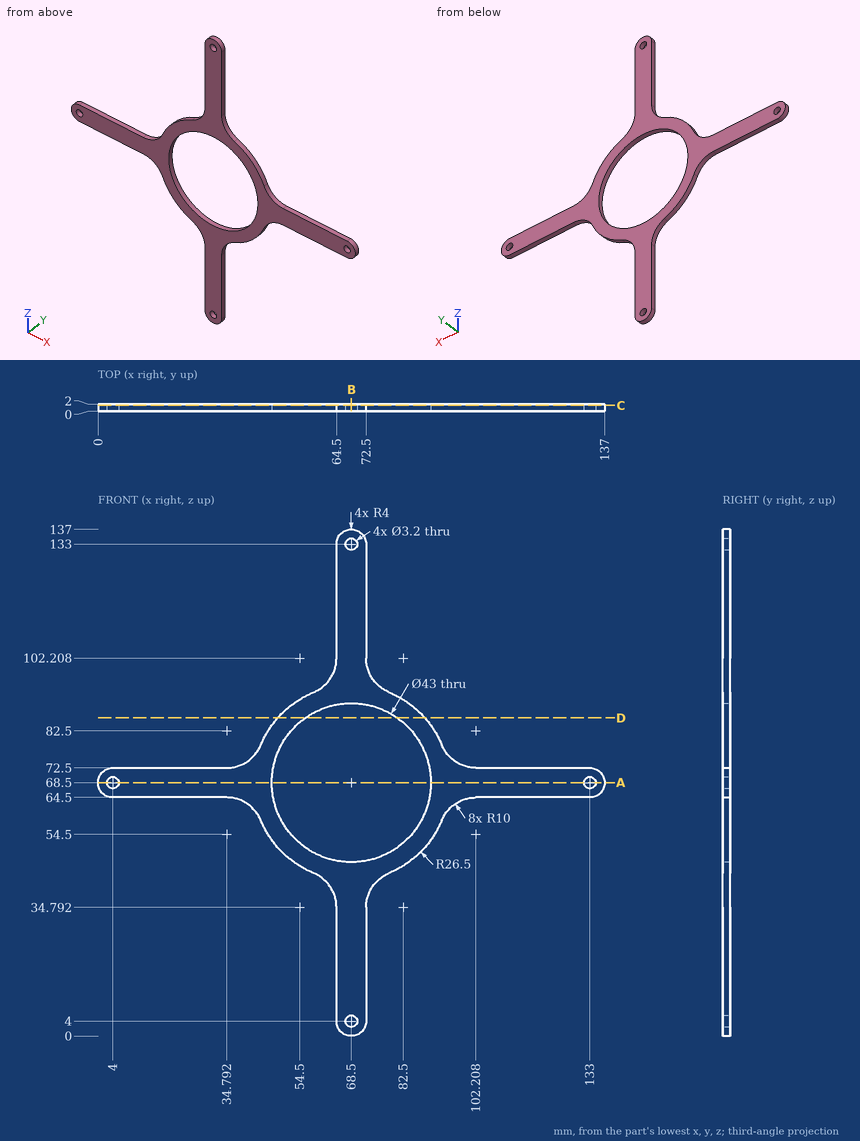
Could you check a few things on this drawing? It's one solid part, dimensions in mm from its lowest x, y, z. Give positions to 0.01 mm unless a question says otherwise; leave off trailing zeros. Loops run counter-clockwise (first coordinate to the right, second up) from the corner with the lowest first, then second, coordinate; pieces in that order, holes last. Notation, with made-up numbers: (24, 85.5) -> (41, 85.5) arc R10 ccw to (41, 102.5) -> close; hole circle Ø7 at (53, 51.5). An arc over 180 degrees is marked (long way). Use one line per item in the form item = value. Start each with the question number.
1) Please list where these lines run through material, in increasing order: line 1 along X through (y, z) = (0.95, 68.5); line 2 along Z through (x, y) = (4, 0.65).
2) Imagine slicing it at D-D (z = 86). Please give me the cut outline in (x, y).
3) Imagine slicing it at A-A (z = 68.5). Please give me the cut outline in (x, y).
4) Imagine slicing it at C-C (y = 1.6). Count the separate pieces of the cut face and the enclosed holes in it, then the cut area to 3 significant figures.
5) Imagine slicing it at B-B (x = 68.5). Please give me the cut outline in (y, z), then the cut area to 3 significant figures.
6) For P1, Ø1, axis at x = 12, y = 1, coming from the +Z side; P2, Ø4, axis at x = 133, z = 68.5, coming from the -Y side; P3, Ø1, axis at y = 1, z = 113.5, coming from the +X side; P4, Ø1, axis at x = 25.5, y = 1.5, coming from the -Z side, each with a flat end and sliding along its axis, tell me the tip position at first contact or that it passes through.
Check values:
q1.line_1 = 0 to 2.4, 5.6 to 47, 90 to 131.4, 134.6 to 137
q1.line_2 = 64.5 to 66.9, 70.1 to 72.5
q2.outline = (48.6, 0) -> (56.01, 0) -> (56.01, 2) -> (48.6, 2) -> close; (80.99, 0) -> (88.4, 0) -> (88.4, 2) -> (80.99, 2) -> close
q3.outline = (0, 0) -> (2.4, 0) -> (2.4, 2) -> (0, 2) -> close; (5.6, 0) -> (47, 0) -> (47, 2) -> (5.6, 2) -> close; (90, 0) -> (131.4, 0) -> (131.4, 2) -> (90, 2) -> close; (134.6, 0) -> (137, 0) -> (137, 2) -> (134.6, 2) -> close
q4.separate_pieces = 1
q4.enclosed_holes = 5
q4.area = 2,120 mm^2
q5.outline = (0, 0) -> (2, 0) -> (2, 2.4) -> (0, 2.4) -> close; (0, 5.6) -> (2, 5.6) -> (2, 47) -> (0, 47) -> close; (0, 90) -> (2, 90) -> (2, 131.4) -> (0, 131.4) -> close; (0, 134.6) -> (2, 134.6) -> (2, 137) -> (0, 137) -> close
q5.area = 175 mm^2
q6.P1 = 72.5
q6.P2 = 0
q6.P3 = 72.5
q6.P4 = 64.5
